The model under review builds one solid part; all positions refer to its coordinate system, in mm. A direction names the side the tool comes from. Coordinates: 2 decimals unless noted, no trailing zeros. Write each loop counter-clockwise with the first axis right and the second up, starting at its lowest first coordinate (ties: lowest second). Pieces come first, ordered by that corner, then holes. Notation, with made-up numbers: (62, -14) - (73, -14) arc R21 cw to (73, 5) - close; hole circle Ø6 at (-31.5, 78.25). An arc over 180 degrees is marked (long way). Return JSON: item names as keys, results as strings. Group by question number.
(1) We need section A-A on x = 0. Give the number of separate pieces and of enclosed holes in the cut face, then the cut area to 3 significant figures.
(2) Tool access review of faces 1 (the face through (-0.31, 4.83, -2.36)), 2 (the face through (2.04, 9.39, -4.93)): name each direction out of +Z, -Z, +X, -X, +Y, -Y from which nothing blocks a thin tool from reaching the whole face with its end or side.
(3) For pin 1 Ø3.5 at (x, y) = (0, 15.621) entering from +Z; pin 2 Ø0.6 at (x, y) = (2, 15.5) entering from +Z; pin 3 Ø5 at (x, y) = (3, 15.5) entering from -Z, all flat-tipped, find the tip position at first contact; note any pin that passes through.
(4) We need section D-D on x = -4.25. State the section outline as (y, z) points.
(5) To check wall thickness, follow L1, parallel to Y at x = -0.75, z = 3; L2, parallel to X at y = 1.75, z = 0.25; L3, parallel to X at y = 3.25, z = 2.5. State the ranges of each line that lie inside material, in increasing order. Write a range as from..to.
(6) Draft analysis for pull direction Y (two halves, no side actions). For faces 3 (the face through (-1.3, 19.05, -1.1)), 4 (the face through (-1.6, 14.39, 2.63)), 5 (the face through (1.1, 0, -2.3)), 6 (the face through (-1.6, 2.2, 3.3)), state which applies: released by +Y, released by -Y, zero draft, split by the parting line, or undercut.
(7) We need section C-C on z = -3.75. State the section outline as (x, y) points, then the cut area to 3 significant figures.
(8) We need section B-B on y = 6.75. State the section outline as (x, z) points, then the cut area to 3 significant figures.
```python
from build123d import *

# Parameters (mm, degrees)
SKETCH1_R                       = 5.334
BOSS_EXTRUDE1_DEPTH             = 19.05
F_3_0MM_DOWEL_HOLE3_D           = 3
F_3_0MM_DOWEL_HOLE3_DEPTH       = 9.525
F_3_0MM_DOWEL_HOLE3_TIP         = 0.901290929
F_3_16_0_1875_DOWEL_HOLE1_D     = 4.7625
F_3_16_0_1875_DOWEL_HOLE1_DEPTH = 9.525
F_3_16_0_1875_DOWEL_HOLE1_TIP   = 1.430799349
F_10_32_TAPPED_HOLE1_OUTLINE_R  = 2.0193
F_10_32_TAPPED_HOLE1_DEPTH      = 6


with BuildPart() as part:
    # Sketch1 → Boss-Extrude1 (new body)
    with BuildSketch(Plane(origin=(0, 0, 0), x_dir=(1, 0, 0), z_dir=(0, 1, 0))):
        with Locations(Location((0, 0, 0), (0, 0, 90))):
            Circle(SKETCH1_R)
    extrude(amount=BOSS_EXTRUDE1_DEPTH)

    # Ø3.0mm Dowel Hole3
    with Locations(Plane(origin=(0, 19.05, 0), x_dir=(1, 0, 0), z_dir=(0, 1, 0))):
        with Locations((0, 0)):
            Hole(F_3_0MM_DOWEL_HOLE3_D / 2, depth=F_3_0MM_DOWEL_HOLE3_DEPTH)
            with Locations((0, 0, -(F_3_0MM_DOWEL_HOLE3_DEPTH + F_3_0MM_DOWEL_HOLE3_TIP / 2))):  # 118° drill point
                Cone(0, F_3_0MM_DOWEL_HOLE3_D / 2, F_3_0MM_DOWEL_HOLE3_TIP, mode=Mode.SUBTRACT)

    # 3/16 (0.1875) Dowel Hole1
    with Locations(Plane(origin=(0, 0, 0), x_dir=(-1, 0, 0), z_dir=(0, -1, 0))):
        with Locations((0, 0)):
            Hole(F_3_16_0_1875_DOWEL_HOLE1_D / 2, depth=F_3_16_0_1875_DOWEL_HOLE1_DEPTH)
            with Locations((0, 0, -(F_3_16_0_1875_DOWEL_HOLE1_DEPTH + F_3_16_0_1875_DOWEL_HOLE1_TIP / 2))):  # 118° drill point
                Cone(0, F_3_16_0_1875_DOWEL_HOLE1_D / 2, F_3_16_0_1875_DOWEL_HOLE1_TIP, mode=Mode.SUBTRACT)

    # #10-32 Tapped Hole1: read off the stored shape, not the designer's step
    # #10-32 Tapped Hole1 outline → #10-32 Tapped Hole1 (cut)
    with BuildSketch(Plane.XY):
        with Locations((0, 3.429)):
            Circle(F_10_32_TAPPED_HOLE1_OUTLINE_R)
        with Locations((0, 15.621)):
            Circle(F_10_32_TAPPED_HOLE1_OUTLINE_R)
    extrude(amount=F_10_32_TAPPED_HOLE1_DEPTH, mode=Mode.SUBTRACT)


solid = part.part
```
Ans:
{
 "1": {"separate pieces": "4", "enclosed holes": "0", "area": "101 mm²"},
 "2": {"face 1": "-Y", "face 2": "+Y, -Y"},
 "3": {"pin 1": "z = 0", "pin 2": "z = 4.95", "pin 3": "z = -5.31"},
 "4": {"outline": "(0, -3.22) - (19.05, -3.22) - (19.05, 3.22) - (0, 3.22) - close"},
 "5": {"L1": "0..1.55, 5.3..13.75, 17.5..19.05", "L2": "-5.33..-2.37, 2.37..5.33", "L3": "-4.71..-2.01, 2.01..4.71"},
 "6": {"face 3": "released by +Y", "face 4": "undercut", "face 5": "released by -Y", "face 6": "undercut"},
 "7": {"outline": "(-3.79, 0) - (3.79, 0) - (3.79, 19.05) - (-3.79, 19.05) - close", "area": "145 mm²"},
 "8": {"outline": "circle Ø10.67 at (0, 0); hole circle Ø4.76 at (0, 0)", "area": "71.6 mm²"}
}
